Read the model definition and answer for the solid it produces. Units are mm, in the model's axes. Face numbers are marked on the shaded views. A direction names the side the tool comes from. Round coordinates to 2 decimals unless told otherwise and drop trailing zeros. Order: outer loops, then holes, each group sorted by start corner. A loop starts at its lowest first (then second) coordinate and runs counter-clockwise, first axis right, second up. Notation, with made-up numbers: (75.5, 28.25) -> (105.5, 28.25) arc R26 ccw to (105.5, 66.25) -> close; hole circle Ø9 at (8.25, 20.25). An arc over 180 degrees is marked (long way). Use a Markdown table: item, result. Add a question column.
1. Section C-C, the plane y = 11 is taken. Give the vertices of the cut face in (x, z).
2. For the marked faces 5 and 6, determine the directions among +Z, -Z, +X, -X, +Y, -Y from which every point of the face is accessible in a straight line to the end or side of a thin tool.
3. Given pin 1 (7 mm diameter, centred on y = 24.3, z = 0, fed in from +X); pin 2 (2.5 mm diameter, centred on y = 25.45, z = 15, fed in from +X); pin 3 (3 mm diameter, centred on x = -11.7, z = -14, fed in from -Y); pin 4 (7 mm diameter, centred on y = 25.45, z = -15, fed in from -X), each flat-ended and moving along its own axis, determine where each tip first touches the part or whether it passes through.
4. Section B-B, the plane x = 11.7 is taken. Give the vertices of the cut face in (y, z), then the cut area to 3 significant figures.
5. Consider L1, parallel to X at y = 35.05, z = -14; L2, parallel to X at y = 11, z = -14; L3, parallel to X at y = 22, z = 0. Determine where each line is inside the solid, lowest interval first. Write a range as [from, to].
6. Section D-D, the plane x = -24 is taken. Give the vertices of the cut face in (y, z), then the cut area to 3 significant figures.
7. The mould has two halves that part along X. Classify the marked faces 1, 2, 3 and 4: +X half, -X half, draft (parallel to the pull), parting line (faces both ways), or undercut.
8. Section A-A, the plane z = -24.5 is taken. Give the vertices of the cut face in (x, y).
```python
from build123d import *

# Parameters (mm, degrees)
SKETCH1_W                      = 54
SKETCH1_H                      = 37.8
BOSS_EXTRUDE1_DEPTH            = 30
SKETCH2_W                      = 42
SKETCH2_H                      = 31.8
CUT_EXTRUDE1_DEPTH             = 76.88043226
CBORE_FOR_M4_SHCS1_D           = 4.5
CBORE_FOR_M4_SHCS1_DEPTH       = 6
CBORE_FOR_M4_SHCS1_CBORE_D     = 8
CBORE_FOR_M4_SHCS1_CBORE_DEPTH = 4
M3X0_5_START                   = 31.8
M3X0_5_TAPPED_HOLE_OUTLINE_R   = 1.25
M3X0_5_TAPPED_HOLE_DEPTH       = 6
CHAMFER1_SIZE                  = 10
M5_CLEARANCE_HOLE1_D           = 5.5
M3X0_5_TAPPED_HOLE1_D          = 2.5
M3X0_5_TAPPED_HOLE1_DEPTH      = 6
SKETCH11_R                     = 1.75
CUT_EXTRUDE2_DEPTH             = 76.88043226
FILLET1_R                      = 1


# Read off the part's stored shape, not the designer's step: M3x0.5 Tapped Hole
with BuildPart() as part:
    # Sketch1 → Boss-Extrude1 (new, symmetric)
    with BuildSketch(Plane.XY):
        with Locations((0, 18.9)):
            Rectangle(SKETCH1_W, SKETCH1_H)
    extrude(amount=BOSS_EXTRUDE1_DEPTH, both=True)

    # Sketch2 → Cut-Extrude1 (cut, through all)
    with BuildSketch(Plane.XY.offset(30)):
        with Locations((0, 15.9)):
            Rectangle(SKETCH2_W, SKETCH2_H)
    extrude(amount=-CUT_EXTRUDE1_DEPTH, mode=Mode.SUBTRACT)

    # CBORE for M4 SHCS1
    with Locations(Plane.ZY.offset(27)):
        with Locations((15, 25.45), (0, 24.3), (0, 7.8), (-15, 25.45)):
            cbore_for_m4_shcs1 = CounterBoreHole(CBORE_FOR_M4_SHCS1_D / 2, CBORE_FOR_M4_SHCS1_CBORE_D / 2, CBORE_FOR_M4_SHCS1_CBORE_DEPTH, depth=CBORE_FOR_M4_SHCS1_DEPTH)

    # M3x0.5 Tapped Hole outline → M3x0.5 Tapped Hole (cut)
    with BuildSketch(Plane(origin=(0, 0, 0), x_dir=(1, 0, 0), z_dir=(0, 1, 0)).offset(M3X0_5_START)):
        with Locations((11.7, -14)):
            Circle(M3X0_5_TAPPED_HOLE_OUTLINE_R)
        with Locations((-11.7, 14)):
            Circle(M3X0_5_TAPPED_HOLE_OUTLINE_R)
        with Locations((-11.7, -14)):
            Circle(M3X0_5_TAPPED_HOLE_OUTLINE_R)
        with Locations((11.7, 14)):
            Circle(M3X0_5_TAPPED_HOLE_OUTLINE_R)
    extrude(amount=M3X0_5_TAPPED_HOLE_DEPTH, mode=Mode.SUBTRACT)

    # Chamfer1
    chamfer1_edges = [part.edges().sort_by_distance(p)[0] for p in [
        (24, 0, 30),
        (-24, 0, 30),
    ]]
    chamfer(chamfer1_edges, length=CHAMFER1_SIZE)

    # Mirror1: CBORE for M4 SHCS1 across plane
    add(cbore_for_m4_shcs1.mirror(Plane(origin=(0, 0, 0), x_dir=(0, 0, 1), z_dir=(1, 0, 0))), mode=Mode.SUBTRACT)

    # M5 Clearance Hole1 (through all)
    with Locations(Plane(origin=(27, 0, 0), x_dir=(0, 0, -1), z_dir=(1, 0, 0))):
        with Locations((24.5, 6.8)):
            Hole(M5_CLEARANCE_HOLE1_D / 2)

    # M3x0.5 Tapped Hole1
    with Locations(Plane(origin=(27, 0, 0), x_dir=(0, 0, -1), z_dir=(1, 0, 0))):
        with Locations((24.5, 25.45)):
            Hole(M3X0_5_TAPPED_HOLE1_D / 2, depth=M3X0_5_TAPPED_HOLE1_DEPTH)

    # Sketch11 → Cut-Extrude2 (cut, through all)
    with BuildSketch(Plane(origin=(0, 0, -30), x_dir=(-1, 0, 0), z_dir=(0, 0, -1))):
        with Locations((-19.25, 31.8)):
            Circle(SKETCH11_R)
        with Locations((19.25, 31.8)):
            Circle(SKETCH11_R)
    extrude(amount=-CUT_EXTRUDE2_DEPTH, mode=Mode.SUBTRACT)

    # Fillet1
    fillet1_edges = [part.edges().sort_by_distance(p)[0] for p in [
        (-17.5, 31.8, 0),
        (17.5, 31.8, 0),
    ]]
    fillet(fillet1_edges, radius=FILLET1_R)


solid = part.part
```
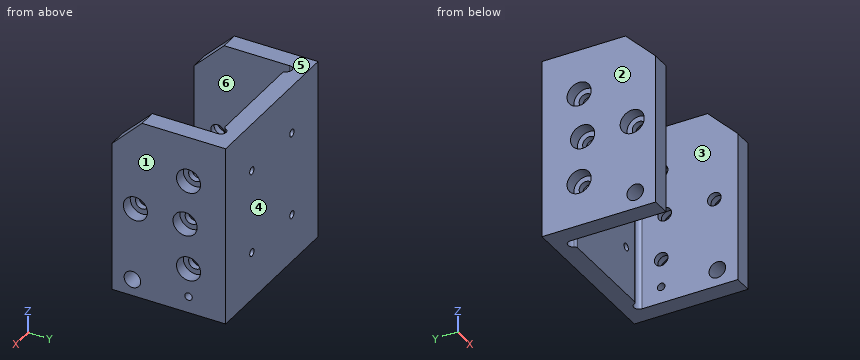
Verdict:
| question | item | result |
|---|---|---|
| 1 | outline | (-27, -30) -> (-21, -30) -> (-21, 30) -> (-27, 30) -> (-27, 2.4) -> (-23, 2.4) -> (-23, -2.4) -> (-27, -2.4) -> close; (21, -30) -> (27, -30) -> (27, -2.4) -> (23, -2.4) -> (23, 2.4) -> (27, 2.4) -> (27, 30) -> (21, 30) -> close |
| 2 | face 5 | +Z, +X, -X, +Y, -Y |
| 2 | face 6 | +Z, -Z, -Y |
| 3 | pin 1 | stops at x = 23 |
| 3 | pin 2 | passes through |
| 3 | pin 3 | stops at y = 31.8 |
| 3 | pin 4 | stops at x = -23 |
| 4 | outline | (31.8, -30) -> (37.8, -30) -> (37.8, -15.25) -> (31.8, -15.25) -> close; (31.8, -12.75) -> (37.8, -12.75) -> (37.8, 12.75) -> (31.8, 12.75) -> close; (31.8, 15.25) -> (37.8, 15.25) -> (37.8, 30) -> (31.8, 30) -> close |
| 4 | area | 330 mm2 |
| 5 | L1 | x = [-27, -12.95], [-10.45, 10.45], [12.95, 27] |
| 5 | L2 | x = [-27, -21], [21, 27] |
| 5 | L3 | x = [-23, -21], [21, 23] |
| 6 | outline | (0, -30) -> (37.8, -30) -> (37.8, 30) -> (10, 30) -> (0, 20) -> close; hole circle Ø8 at (7.8, 0); hole circle Ø5.5 at (6.8, -24.5); hole circle Ø8 at (24.3, 0); hole circle Ø8 at (25.45, -15); hole circle Ø8 at (25.45, 15) |
| 6 | area | 1,990 mm2 |
| 7 | face 1 | +X half |
| 7 | face 2 | -X half |
| 7 | face 3 | undercut |
| 7 | face 4 | draft |
| 8 | outline | (-27, 0) -> (-21, 0) -> (-21, 4.05) -> (-27, 4.05) -> close; (-27, 9.55) -> (-21, 9.55) -> (-21, 31.8) arc R1.75 cw to (-17.62, 32.44) arc R1 ccw to (-16.69, 31.8) -> (16.69, 31.8) arc R1 ccw to (17.62, 32.44) arc R1.75 cw to (21, 31.8) -> (21, 26.7) -> (27, 26.7) -> (27, 37.8) -> (-27, 37.8) -> close; (21, 0) -> (27, 0) -> (27, 4.05) -> (21, 4.05) -> close; (21, 9.55) -> (27, 9.55) -> (27, 24.2) -> (21, 24.2) -> close |
